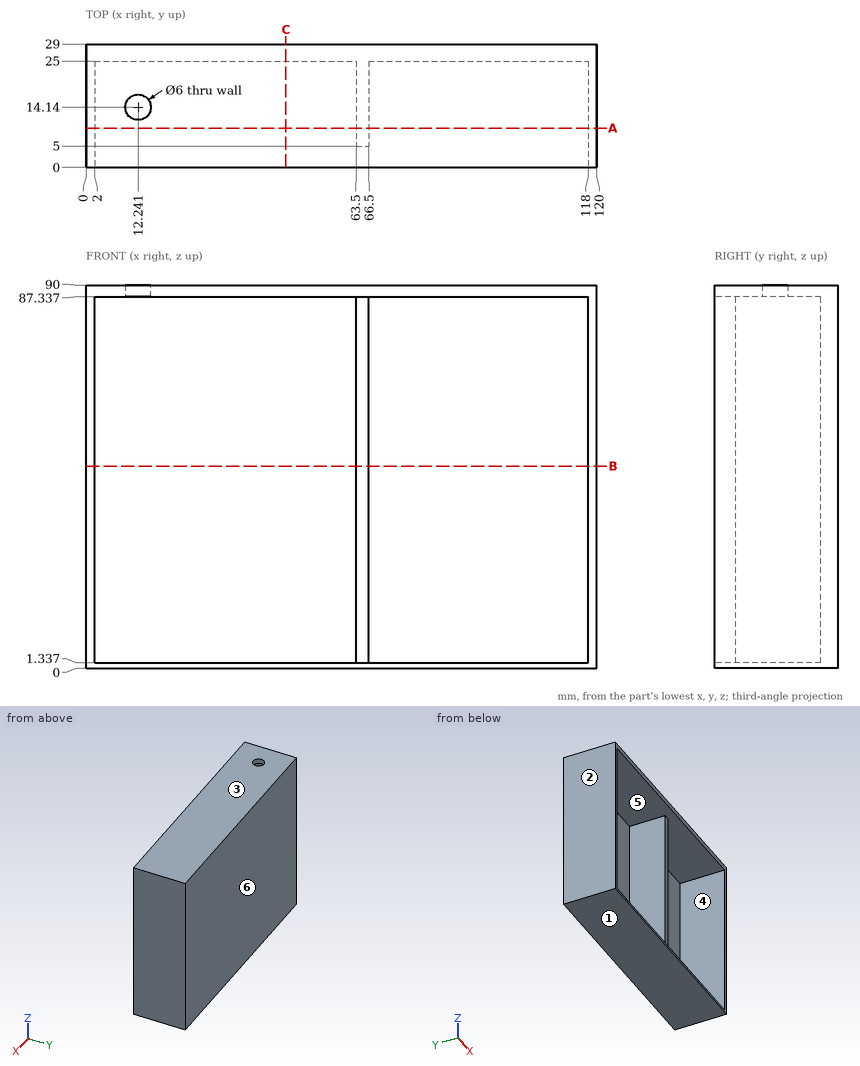
Drawing for the job (mm, zero at the part's lowest x, y, z). A direction names the side the tool comes from. Give positions to 0.01 mm unless a question says otherwise; leave off trailing zeros. Write each loop counter-clockwise with the first axis right and the second up, starting at its lowest first coordinate (ties: lowest second). Pieces come first, ordered by that corner, then holes. Notation, with made-up numbers: (52, 83) -> (100, 83) arc R18 ccw to (100, 118) -> close; hole circle Ø1 at (74, -19). An arc over 180 degrees is marked (long way). Put each result on its own line as item: value. Start each with the question number.
Item 1: Wall check: L1, parallel to X at y = 19.5, z = 19.5; L2, parallel to Z at x = 101, y = 21.25; L3, parallel to X at y = 2, z = 59. Give the ranges that are in metal, low to high. Write a range as [from, to].
Item 2: Pin check, flat tips, straight feed: pin 1 Ø1 at (x, y) = (51, 25.5) entering from -Z; pin 2 Ø15.5 at (x, z) = (95.5, 30) entering from -Y; pin 3 Ø2.5 at (x, z) = (65, 56) entering from -Y. Stop position of each tip, or through.
Item 3: Cut at B-B (z = 47.5). List the corners of the cut face in (x, y).
Item 4: Pull direction Z, two halves, no side cores. Call the marked faces 1, 2, 3 and 4: pulls with the +Z half, pulls with the -Z half, needs draft (parallel to the pull), parting line crosses it, or undercut.
Item 5: Cut at A-A (y = 9.25). List the corners of the cut face in (x, z).
Item 6: Cut at C-C (x = 47). List the corners of the cut face in (y, z).
Item 7: Which spindle directions (+Z, -Z, +X, -X, +Y, -Y) get a long thin tool onto all of the face, cutting with end or side? Do the marked faces 5 and 6. Say none if no direction does.
Answer list:
1. L1: x = [0, 2], [63.5, 66.5], [118, 120]
1. L2: z = [0, 1.34], [87.34, 90]
1. L3: x = [0, 2], [118, 120]
2. pin 1: stops at z = 0
2. pin 2: stops at y = 25
2. pin 3: stops at y = 5
3. outline: (0, 0) -> (2, 0) -> (2, 25) -> (63.5, 25) -> (63.5, 5) -> (66.5, 5) -> (66.5, 25) -> (118, 25) -> (118, 0) -> (120, 0) -> (120, 29) -> (0, 29) -> close
4. face 1: pulls with the -Z half
4. face 2: needs draft
4. face 3: pulls with the +Z half
4. face 4: undercut
5. outline: (0, 0) -> (120, 0) -> (120, 90) -> (0, 90) -> close; hole (2, 1.34) -> (63.5, 1.34) -> (63.5, 87.34) -> (2, 87.34) -> close; hole (66.5, 1.34) -> (118, 1.34) -> (118, 87.34) -> (66.5, 87.34) -> close
6. outline: (0, 0) -> (29, 0) -> (29, 90) -> (0, 90) -> (0, 87.34) -> (25, 87.34) -> (25, 1.34) -> (0, 1.34) -> close
7. face 5: -Y
7. face 6: +Z, -Z, +X, -X, +Y
